Verification items for this drawing (mm, ordinates from the low corner). Round coordinates to 2 decimals unless told otherwise and drop trailing zeros. Order: outer loops, then holes, each group sorted by start corner. A loop starts at its lowest first (then second) coordinate and runs counter-clockwise, first axis right, second up.
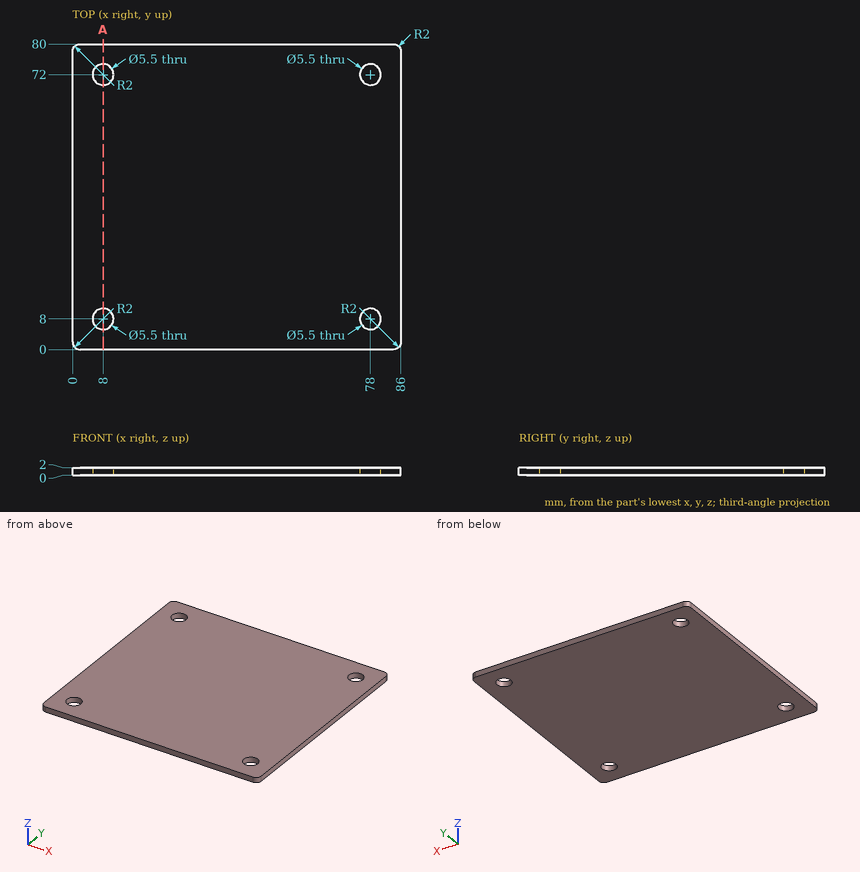
Item 1: Sectioned sample at A-A (x = 8). Record the cut outline in (y, z).
Answer:
outline: (0, 0) - (5.25, 0) - (5.25, 2) - (0, 2) - close; (10.75, 0) - (69.25, 0) - (69.25, 2) - (10.75, 2) - close; (74.75, 0) - (80, 0) - (80, 2) - (74.75, 2) - close
Item 2: Go/stop test with a flat-tipped pin: P1, Ø5, axis at x = 8, y = 72, coming from the -Z side. Record where the tip stops, or that it passes through.
Answer:
P1: passes through
Item 3: Scan lines: line 1 along Y through (x, z) = (8, 0.65); line 2 along Y through (x, z) = (80, 1.4); line 3 along X through (y, z) = (7, 1.6). Record each from-to range of solid material in increasing order.
Answer:
line 1: y = 0 to 5.25, 10.75 to 69.25, 74.75 to 80
line 2: y = 0 to 6.11, 9.89 to 70.11, 73.89 to 80
line 3: x = 0 to 5.44, 10.56 to 75.44, 80.56 to 86
